Here's how the part is built. I have some questions about the finished solid (model axes, mm). A direction names the side the tool comes from. Coordinates: 2 decimals unless noted, no trailing zeros. Loops run counter-clockwise (first coordinate to the right, second up) from the corner with the lowest first, then second, coordinate; pieces in that order, holes last. Notation, with made-up numbers: M -35,-12 L 19,-12 A20 ccw 19,1 Z; hole C -39,43 d2. An arc over 180 degrees is marked long. Use CSV: the item, a comma, the result in double quotes. Start each with the question number.
Q1. Which directions (+Z, -Z, +X, -X, +Y, -Y) give clear straight access to the entire face, cutting with the end or side of a thin tool? Please do faces 1 (the flat face through (-19.45, 10, 0)), 2 (the cylindrical face through (-14.65, 12.8, 0.09)).
Q2. If we section it at D-D (z = 2): Please give me the cut outline in (x, y), and give its area (3 significant figures).
Q3. Please list where these lines run through material, in increasing order: probe 1 along X at (y, z) = (15, 1); probe 2 along X at (y, z) = (7, 4.5); probe 3 along Y at (x, z) = (-11, 5.75). Write a range as [from, to].
Q4. If we section it at B-B (z = 0): Please give me the cut outline in (x, y).
Q5. If we section it at C-C (x = -3): Please give me the cut outline in (y, z).
Q6. If we section it at A-A (y = 11): Please give me the cut outline in (x, z), and give its area (3 significant figures).
Q7. If we mould it in two halves opening along Z, with no side actions, what happens to faces 3 (the flat face through (-17, 20, 0)), 4 (the cylindrical face through (14.65, 12.8, -0.09)), 5 (the flat face through (0, 5, 6.4))? For each: +Z half, -Z half, draft (parallel to the pull), parting line (faces both ways), or undercut.
from build123d import *

# Parameters (mm, degrees)
SKETCH2_W           = 38.9
SKETCH2_H           = 12.8
BOSS_EXTRUDE1_DEPTH = 5.8
SKETCH3_R           = 6.4
BOSS_EXTRUDE2_DEPTH = 14.2


with BuildPart() as part:
    # Sketch2 → Boss-Extrude1 (new body)
    with BuildSketch(Plane(origin=(0, 0, 0), x_dir=(1, 0, 0), z_dir=(0, 1, 0))):
        Rectangle(SKETCH2_W, SKETCH2_H)
    extrude(amount=BOSS_EXTRUDE1_DEPTH)

    # Sketch3 → Boss-Extrude2 (add)
    with BuildSketch(Plane(origin=(0, 5.8, 0), x_dir=(1, 0, 0), z_dir=(0, 1, 0))):
        with BuildLine():
            Line((-13.178106844, 6.4), (-19.45, 6.4))
            Line((-19.45, 6.4), (-19.45, -6.4))
            Line((-19.45, -6.4), (-13.178106844, -6.4))
            ThreePointArc((-13.178106844, -6.4), (-14.65, 0), (-13.178106844, 6.4))
        make_face()
        Circle(SKETCH3_R)
        with BuildLine():
            Line((19.45, 6.4), (13.178106844, 6.4))
            ThreePointArc((13.178106844, 6.4), (14.65, 0), (13.178106844, -6.4))
            Line((13.178106844, -6.4), (19.45, -6.4))
            Line((19.45, -6.4), (19.45, 6.4))
        make_face()
    extrude(amount=BOSS_EXTRUDE2_DEPTH)


solid = part.part
Results below:
1,face 1,"+Z, -Z, -X, +Y, -Y"
1,face 2,"+Y"
2,outline,"M -19.45,0 L 19.45,0 L 19.45,20 L 14.51,20 L 14.51,5.8 L 6.08,5.8 L 6.08,20 L -6.08,20 L -6.08,5.8 L -14.51,5.8 L -14.51,20 L -19.45,20 Z"
2,area,"538 mm^2"
3,probe 1,"[-19.45, -14.62], [-6.32, 6.32], [14.62, 19.45]"
3,probe 2,"[-19.45, -13.94], [-4.55, 4.55], [13.94, 19.45]"
3,probe 3,"[0, 5.8]"
4,outline,"M -19.45,0 L 19.45,0 L 19.45,20 L 14.65,20 L 14.65,5.8 L 6.4,5.8 L 6.4,20 L -6.4,20 L -6.4,5.8 L -14.65,5.8 L -14.65,20 L -19.45,20 Z"
5,outline,"M 0,-6.4 L 5.8,-6.4 L 5.8,-5.65 L 20,-5.65 L 20,5.65 L 5.8,5.65 L 5.8,6.4 L 0,6.4 Z"
6,outline,"M -19.45,-6.4 L -13.18,-6.4 A14.65 cw -13.18,6.4 L -19.45,6.4 Z; C 0,0 d12.8; M 13.18,-6.4 L 19.45,-6.4 L 19.45,6.4 L 13.18,6.4 A14.65 cw Z"
6,area,"264 mm^2"
7,face 3,"draft"
7,face 4,"undercut"
7,face 5,"+Z half"
